Could you check a few things on this drawing? It's one solid part, dimensions in mm from its lowest x, y, z. A direction names the side the tool comes from. Coordinates: 2 decimals unless noted, no trailing zeros. Order: outer loops, then holes, each group sorted by start corner. A loop starts at its lowest first (then second) coordinate and runs counter-clockwise, first axis right, second up. Notation, with made-up numbers: (-22.5, 32.5) -> (9.5, 32.5) arc R9 cw to (9.5, 48.5) -> close; hole circle Ø7 at (76, 69.5). An arc over 180 degrees is marked (long way). Use a Markdown table: item, result. Add a question column.
1. For pin 1 Ø1.9 at (x, y) = (71, 4) entering from +Z; pin 2 Ø5 at (x, y) = (52.5, 28.15) entering from +Z; pin 3 Ø4.5 at (x, z) = (39.5, 14.5) entering from -Y, each with a flat end and sliding along its axis, tell me the tip position at first contact or that it passes through.
2. Suppose I cut it at C-C, the plane z = 4.5. List the corners of the cut face in (x, y) for me, then the cut area to 3 significant figures.
3. Suppose I cut it at A-A, the plane y = 4. List the corners of the cut face in (x, z) for me.
4. Suppose I cut it at D-D, the plane y = 18.15. List the corners of the cut face in (x, z) for me.
5. For the marked faces 4, 5 and 6, which set-ups out of +Z, -Z, +X, -X, +Y, -Y let a thin tool reach every point of the face, with its end or its side?
6. Suppose I cut it at B-B, the plane x = 22. List the corners of the cut face in (y, z) for me, then the cut area to 3 significant figures.
7. If I drill on line 1 along X through (y, z) = (18, 2.75); line 2 along X through (y, z) = (49.5, 17); line 3 along Y through (x, z) = (4.5, 1.85), over which ranges is the centre line in solid material (lowest first)? Write a range as from..to.
8. We'd pull the mould along X, two halves only. Please class the marked faces 1, 2 and 3: pulls with the +X half, pulls with the -X half, needs draft (parallel to the pull), parting line crosses it, or undercut.
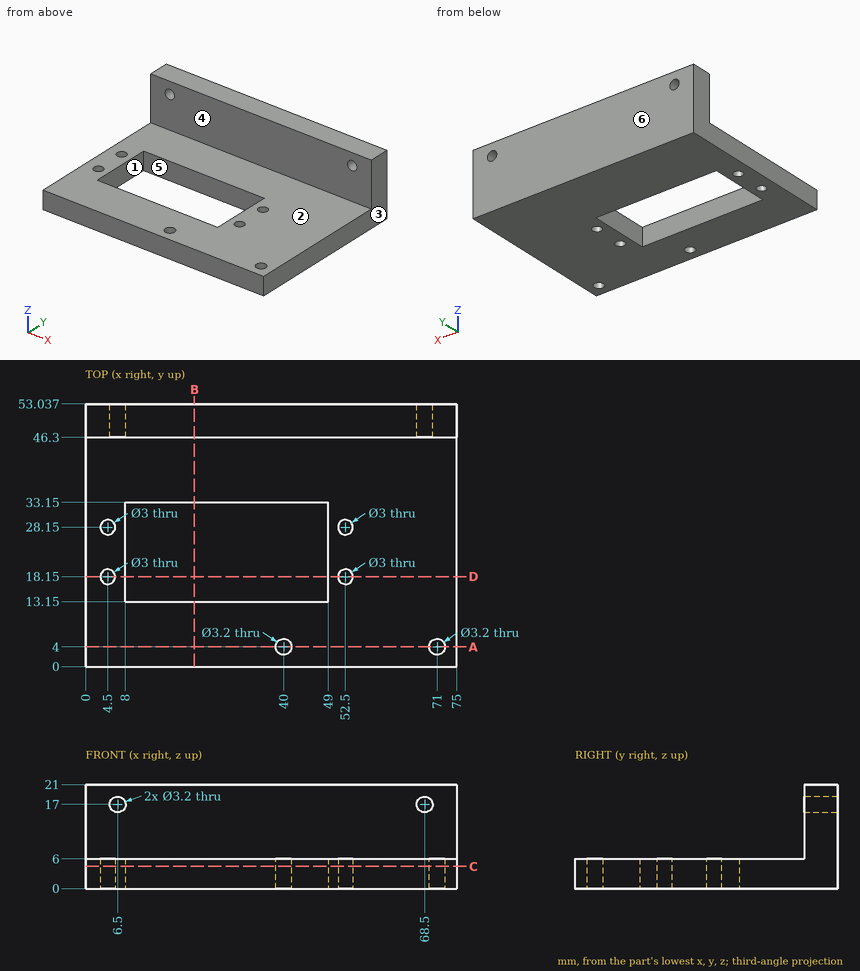
Worked out:
| question | item | result |
|---|---|---|
| 1 | pin 1 | passes through |
| 1 | pin 2 | stops at z = 6 |
| 1 | pin 3 | stops at y = 46.3 |
| 2 | outline | (0, 0) -> (75, 0) -> (75, 53.04) -> (0, 53.04) -> close; hole circle Ø3 at (4.5, 18.15); hole circle Ø3 at (4.5, 28.15); hole (8, 13.15) -> (49, 13.15) -> (49, 33.15) -> (8, 33.15) -> close; hole circle Ø3.2 at (40, 4); hole circle Ø3 at (52.5, 18.15); hole circle Ø3 at (52.5, 28.15); hole circle Ø3.2 at (71, 4) |
| 2 | area | 3,110 mm² |
| 3 | outline | (0, 0) -> (38.4, 0) -> (38.4, 6) -> (0, 6) -> close; (41.6, 0) -> (69.4, 0) -> (69.4, 6) -> (41.6, 6) -> close; (72.6, 0) -> (75, 0) -> (75, 6) -> (72.6, 6) -> close |
| 4 | outline | (0, 0) -> (3, 0) -> (3, 6) -> (0, 6) -> close; (6, 0) -> (8, 0) -> (8, 6) -> (6, 6) -> close; (49, 0) -> (51, 0) -> (51, 6) -> (49, 6) -> close; (54, 0) -> (75, 0) -> (75, 6) -> (54, 6) -> close |
| 5 | face 4 | +Z, +X, -X, -Y |
| 5 | face 5 | +Z, -Z |
| 5 | face 6 | +Z, -Z, +X, -X, +Y |
| 6 | outline | (0, 0) -> (13.15, 0) -> (13.15, 6) -> (0, 6) -> close; (33.15, 0) -> (53.04, 0) -> (53.04, 21) -> (46.3, 21) -> (46.3, 6) -> (33.15, 6) -> close |
| 6 | area | 299 mm² |
| 7 | line 1 | x = 0..3.01, 5.99..8, 49..51.01, 53.99..75 |
| 7 | line 2 | x = 0..4.9, 8.1..66.9, 70.1..75 |
| 7 | line 3 | y = 0..16.65, 19.65..26.65, 29.65..53.04 |
| 8 | face 1 | undercut |
| 8 | face 2 | needs draft |
| 8 | face 3 | pulls with the +X half |
